Can you work these out from the model? Positions are in its coordinate system, mm. Face numbers are marked on the shaded views. A direction names the side the tool comes from. Coordinates: 2 decimals unless noted, no trailing zeros. Order: outer loops, then holes, each group sorted by start corner. A loop starts at its lowest first (then second) coordinate and runs counter-clockwise, first axis right, second up. Notation, with made-up numbers: M -27.5,87.5 L -14.5,87.5 A16 cw -14.5,99.5 Z; hole C 46,84 d4. An arc over 180 degrees is marked long. Answer as CSV lines item,"result". Start each with the question number.
1. Will these pins go through, and if not, where does the flat tip stop? pin 1 (0.9 mm diameter, centred on y = 1, z = 23, fed in from +X); pin 2 (1.4 mm diameter, centred on x = 1.5, y = 2, fed in from +Z); pin 3 (0.9 mm diameter, centred on y = 2, z = 23.5, fed in from -X).
2. If we section it at C-C (x = 8.25): List the corners of the cut face in (y, z) for me, plus the area to 3 significant figures.
3. If we section it at B-B (y = 1.85): List the corners of the cut face in (x, z) for me, plus the area to 3 significant figures.
4. I need wall thicknesses on line 1 along X through (y, z) = (1.2, 0); line 2 along Z through (x, y) = (5.25, 2.1); line 3 along Z through (x, y) = (4.25, 1.8). Which ranges of each line are inside material? Lowest first, please. Write a range as from..to.
5. On a 3-axis mill with a long thin cutter (end or side, diameter ignored), from which of +Z, -Z, +X, -X, +Y, -Y can I reach the whole of each face in a straight line? I mean the marked faces 1, 2 and 3. Say none if no direction works.
6. If we section it at A-A (x = 5.25): List the corners of the cut face in (y, z) for me, plus the area to 4 significant figures.
7. If we section it at D-D (x = 1.25): List the corners of the cut face in (y, z) for me.
8. If we mould it in two halves opening along Z, with no side actions, what happens to the marked faces 4, 5 and 6? For each: released by +Z, released by -Z, zero draft, split by the parting line, or undercut.
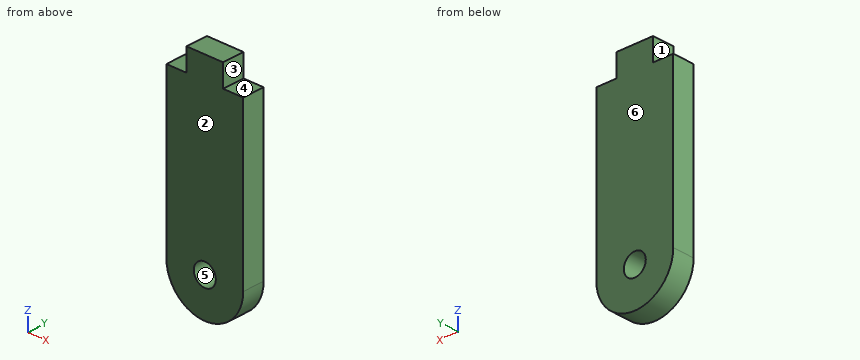
```python
from build123d import *

# Parameters (mm, degrees)
SKETCH_1_W      = 5
SKETCH_1_H      = 3
EXTRUDE_1_DEPTH = 3


with BuildPart() as part:
    # 草图1 → 凸台-拉伸1 (new body)
    with BuildSketch(Plane(origin=(0, 0, 0), x_dir=(1, 0, 0), z_dir=(0, 1, 0))):
        with BuildLine():
            Line((10.5, -22), (10.5, 0))
            ThreePointArc((10.5, 0), (5.25, -5.25), (0, 0))
            Line((0, 0), (0, -22))
            Line((0, -22), (2.75, -22))
            Line((2.75, -22), (7.75, -22))
            Line((7.75, -22), (10.5, -22))
        make_face()
        with Locations((5.25, -23.5)):
            Rectangle(SKETCH_1_W, SKETCH_1_H)
        with BuildLine():
            ThreePointArc((3.75, 0), (5.25, 1.5), (6.75, 0))
            Line((6.75, 0), (10.5, 0))
            ThreePointArc((10.5, 0), (5.25, 5.25), (0, 0))
            Line((0, 0), (3.75, 0))
        make_face()
        with BuildLine():
            Line((10.5, 0), (6.75, 0))
            ThreePointArc((6.75, 0), (5.25, -1.5), (3.75, 0))
            Line((3.75, 0), (0, 0))
            ThreePointArc((0, 0), (5.25, -5.25), (10.5, 0))
        make_face()
    extrude(amount=EXTRUDE_1_DEPTH)


solid = part.part
```
Solved:
1,pin 1,"x = 7.75"
1,pin 2,"z = 22"
1,pin 3,"x = 2.75"
2,outline,"M 0,-4.31 L 3,-4.31 L 3,22 L 0,22 Z"
2,area,"78.9 mm²"
3,outline,"M 0,0 A5.25 ccw 10.5,0 L 10.5,22 L 7.75,22 L 7.75,25 L 2.75,25 L 2.75,22 L 0,22 Z; hole C 5.25,0 d3"
3,area,"282 mm²"
4,line 1,"0..3.75, 6.75..10.5"
4,line 2,"-5.25..-1.5, 1.5..25"
4,line 3,"-5.15..-1.12, 1.12..25"
5,face 1,"+Z, -X, +Y, -Y"
5,face 2,"+Z, -Z, +X, -X, -Y"
5,face 3,"+Z, +X, +Y, -Y"
6,outline,"M 0,-5.25 L 3,-5.25 L 3,-1.5 L 0,-1.5 Z; M 0,1.5 L 3,1.5 L 3,25 L 0,25 Z"
6,area,"81.75 mm²"
7,outline,"M 0,-3.4 L 3,-3.4 L 3,22 L 0,22 Z"
8,face 4,"released by +Z"
8,face 5,"undercut"
8,face 6,"zero draft"
